from build123d import *

# Parameters (mm, degrees)
BOSS_EXTRUDE1_DEPTH = 5
BOSS_EXTRUDE2_DEPTH = 30
SKETCH3_W           = 60
SKETCH3_H           = 61
CUT_EXTRUDE1_DEPTH  = 162.957556168


with BuildPart() as part:
    # Sketch1 → Boss-Extrude1 (new body)
    with BuildSketch(Plane(origin=(0, 0, 0), x_dir=(1, 0, 0), z_dir=(0, 1, 0))):
        Polygon((67.5, -50), (45, -50), (45, -143), (-45, -143), (-45, -50), (-67.5, -50), (-67.5, 50), (67.5, 50), align=None)
    extrude(amount=BOSS_EXTRUDE1_DEPTH)

    # Sketch2 → Boss-Extrude2 (add)
    with BuildSketch(Plane(origin=(0, 5, 0), x_dir=(1, 0, 0), z_dir=(0, 1, 0))):
        Polygon((-67.5, 50), (-67.5, -50), (-45, -50), (-45, -143), (45, -143), (45, -50), (67.5, -50), (67.5, 50), align=None)
        Polygon((52.5, 35), (-52.5, 35), (-52.5, -35), (-30, -35), (-30, -128), (30, -128), (30, -35), (52.5, -35), align=None, mode=Mode.SUBTRACT)
    extrude(amount=BOSS_EXTRUDE2_DEPTH)

    # Sketch3 → Cut-Extrude1 (cut, through all)
    with BuildSketch(Plane(origin=(0, 35, 0), x_dir=(1, 0, 0), z_dir=(0, 1, 0))):
        with Locations((0, -112.5)):
            Rectangle(SKETCH3_W, SKETCH3_H)
    extrude(amount=-CUT_EXTRUDE1_DEPTH, mode=Mode.SUBTRACT)


solid = part.part
The model under review builds one solid part; all positions refer to its coordinate system, in mm. A direction names the side the tool comes from. Coordinates: 2 decimals unless noted, no trailing zeros. Write each loop counter-clockwise with the first axis right and the second up, starting at its lowest first coordinate (ties: lowest second). Pieces come first, ordered by that corner, then holes. Notation, with made-up numbers: (-15, -27) - (23, -27) arc R28 ccw to (23, 6) - close; hole circle Ø3 at (13, -39). An arc over 180 degrees is marked (long way). Answer as a JSON object with one key per item and string values. Group by question number.
1. Add section A-A (z = 92.5). Give the boundary of the cut face in (x, y), plus the area to 3 significant figures.
2. Machinability: for faces 1 (the face through (-45, 17, 96)), 2 (the face through (30, 18, 90)), 3 (the face through (41, 20, 35)), 4 (the face through (0, 3, 82)), which of the approach directions +Z, -Z, +X, -X, +Y, -Y give a long, thin tool a straight path to every point of the face, cutting with its end or side? Answer none if there is none.
3. To check wall thickness, follow probe 1 along Z at (x, y) = (-37, 17); probe 2 along X at (y, z) = (3, 93); probe 3 along X at (y, z) = (31.5, -24). State the ranges of each line that lie inside material, in increasing order.
4. Add section D-D (z = 52). Give the boundary of the cut face in (x, y), plus the area to 3 significant figures.
5. Mouldability with a two-part tool opening along X and no side actions: class faces 5 (the face through (-41, 20, 35)), 6 (the face through (-67.5, 17, -1)), 7 (the face through (1, 20, -35)), 8 (the face through (37, 17, 143)) as pulls with the +X half, pulls with the -X half, needs draft (parallel to the pull), parting line crosses it, or undercut.
6. Clearance check with flat-ended pins moving along their axes: pin 1 Ø6 at (x, y) = (14, 17) entering from +Z; pin 2 Ø3 at (y, z) = (5, 79) entering from +X; pin 3 Ø7 at (x, y) = (-59, 23) entering from +Z. State where each tip first meets the part, or that it passes through.
7. Add section C-C (y = 28.5). Give the boundary of the cut face in (x, z), plus the area to 3 significant figures.
8. Add section B-B (x = 19). Give the boundary of the cut face in (y, z).
Findings:
{
 "1": {"outline": "(-45, 0) - (-30, 0) - (-30, 35) - (-45, 35) - close; (30, 0) - (45, 0) - (45, 35) - (30, 35) - close", "area": "1,050 mm²"},
 "2": {"face 1": "+Z, -X, +Y, -Y", "face 2": "+Z, +Y", "face 3": "+Y", "face 4": "+Z, +Y, -Y"},
 "3": {"probe 1": "-50 to -35, 35 to 143", "probe 2": "-45 to -30, 30 to 45", "probe 3": "-67.5 to -52.5, 52.5 to 67.5"},
 "4": {"outline": "(-45, 0) - (45, 0) - (45, 35) - (30, 35) - (30, 5) - (-30, 5) - (-30, 35) - (-45, 35) - close", "area": "1,350 mm²"},
 "5": {"face 5": "undercut", "face 6": "pulls with the -X half", "face 7": "undercut", "face 8": "needs draft"},
 "6": {"pin 1": "z = -35", "pin 2": "x = 45", "pin 3": "z = 50"},
 "7": {"outline": "(-67.5, -50) - (67.5, -50) - (67.5, 50) - (45, 50) - (45, 143) - (30, 143) - (30, 35) - (52.5, 35) - (52.5, -35) - (-52.5, -35) - (-52.5, 35) - (-30, 35) - (-30, 143) - (-45, 143) - (-45, 50) - (-67.5, 50) - close", "area": "8,040 mm²"},
 "8": {"outline": "(0, -50) - (35, -50) - (35, -35) - (5, -35) - (5, 82) - (0, 82) - close"}
}
